Source: CAD feature listing. Evaluate the final solid. Frame: model axes, mm. A direction names the side the tool comes from. Give positions to 0.01 mm unless a question says otherwise; leave off trailing zeros. Loops run counter-clockwise (first coordinate to the right, second up) from the corner with the lowest first, then second, coordinate; pieces in that order, holes last. Notation, with made-up numbers: M 53.25,55.5 L 89.25,55.5 A15 ccw 89.25,59.5 Z; hole C 11,-4 d4. An arc over 180 degrees is marked long. Answer in a Markdown table with one row per item.
```python
from build123d import *

# Parameters (mm, degrees)
SKETCH3_W             = 20.066
SKETCH3_H             = 20.066
BOSS_EXTRUDE1_DEPTH   = 4.7625
SKETCH6_R             = 8.5725
CUT_EXTRUDE4_DEPTH    = 5.7625
SKETCH61_R            = 8.5725
CUT_EXTRUDE41_DEPTH   = 5.7625
SKETCH62_R            = 9.525
CUT_EXTRUDE42_DEPTH   = 5.7625
F_6_CLEARANCE_HOLE1_D = 4.3053
CUT_EXTRUDE43_REACH   = 6.763
FILLET1_R             = 1.5875


with BuildPart() as part:
    # Sketch3 → Boss-Extrude1 (new body)
    with BuildSketch(Plane.XY):
        with BuildLine():
            Line((-0.5715, -189.484), (41.8465, -189.484))
            ThreePointArc((41.8465, -189.484), (42.969032015, -189.019032015), (43.434, -187.8965))
            Line((43.434, -187.8965), (43.434, -183.134))
            ThreePointArc((43.434, -183.134), (45.293871939, -178.643871939), (49.784, -176.784))
            Line((49.784, -176.784), (54.5465, -176.784))
            ThreePointArc((54.5465, -176.784), (55.669032015, -176.319032015), (56.134, -175.1965))
            Line((56.134, -175.1965), (56.134, -72.4535))
            ThreePointArc((56.134, -72.4535), (55.669032015, -71.330967985), (54.5465, -70.866))
            Line((54.5465, -70.866), (49.784, -70.866))
            ThreePointArc((49.784, -70.866), (45.293871939, -69.006128061), (43.434, -64.516))
            Line((43.434, -64.516), (43.434, -59.7535))
            ThreePointArc((43.434, -59.7535), (42.969032015, -58.630967985), (41.8465, -58.166))
            Line((41.8465, -58.166), (32.3215, -58.166))
            ThreePointArc((32.3215, -58.166), (31.198967985, -57.701032015), (30.734, -56.5785))
            Line((30.734, -56.5785), (30.734, -13.7795))
            ThreePointArc((30.734, -13.7795), (30.269032015, -12.656967985), (29.1465, -12.192))
            Line((29.1465, -12.192), (-54.5465, -12.192))
            ThreePointArc((-54.5465, -12.192), (-55.669032015, -12.656967985), (-56.134, -13.7795))
            Line((-56.134, -13.7795), (-56.134, -140.9065))
            ThreePointArc((-56.134, -140.9065), (-55.669032015, -142.029032015), (-54.5465, -142.494))
            Line((-54.5465, -142.494), (-3.7465, -142.494))
            ThreePointArc((-3.7465, -142.494), (-2.623967985, -142.958967985), (-2.159, -144.0815))
            Line((-2.159, -144.0815), (-2.159, -187.8965))
            ThreePointArc((-2.159, -187.8965), (-1.694032015, -189.019032015), (-0.5715, -189.484))
        make_face()
        with Locations((23.8125, -158.75)):
            Rectangle(SKETCH3_W, SKETCH3_H, mode=Mode.SUBTRACT)
    extrude(amount=BOSS_EXTRUDE1_DEPTH)

    # Sketch6 → Cut-Extrude4 (cut, through all)
    with BuildSketch(Plane(origin=(161.486140968, -518.011138809, 4.7625), x_dir=(1, 0, 0), z_dir=(0, 0, 1))):
        with Locations((-137.673640968, 421.491138809)):
            Circle(SKETCH6_R)
    extrude(amount=-CUT_EXTRUDE4_DEPTH, mode=Mode.SUBTRACT)

    # Sketch61 → Cut-Extrude41 (cut, through all)
    with BuildSketch(Plane(origin=(147.833640968, -456.416138809, 4.7625), x_dir=(1, 0, 0), z_dir=(0, 0, 1))):
        with Locations((-137.673640968, 421.491138809)):
            Circle(SKETCH61_R)
    extrude(amount=-CUT_EXTRUDE41_DEPTH, mode=Mode.SUBTRACT)

    # Sketch62 → Cut-Extrude42 (cut, through all)
    with BuildSketch(Plane.XY.offset(4.7625)):
        with Locations((-37.592, -116.078)):
            Circle(SKETCH62_R)
    extrude(amount=-CUT_EXTRUDE42_DEPTH, mode=Mode.SUBTRACT)

    # #6 Clearance Hole1 (through all)
    with Locations(Plane(origin=(36.5125, -265.1125, 6.35), x_dir=(-1, 0, 0), z_dir=(0, 0, 1))):
        with Locations((49.4665, -130.4925), (-12.7, -136.525), (46.1645, -240.9825)):
            Hole(F_6_CLEARANCE_HOLE1_D / 2)

    # Sketch67 → Cut-Extrude43 (cut, up to next)
    with BuildSketch(Plane(origin=(0, 0, 0), x_dir=(-1, 0, 0), z_dir=(0, 0, -1)), mode=Mode.PRIVATE) as cut_extrude43_sk1:
        with BuildLine():
            Line((-19.558, -170.65625), (-19.558, -167.48125))
            ThreePointArc((-19.558, -167.48125), (-16.66875, -164.592), (-13.7795, -167.48125))
            Line((-13.7795, -167.48125), (-13.7795, -170.65625))
            ThreePointArc((-13.7795, -170.65625), (-16.66875, -173.5455), (-19.558, -170.65625))
        make_face()
    cut_extrude43_tool1 = extrude(cut_extrude43_sk1.sketch, amount=-CUT_EXTRUDE43_REACH, mode=Mode.PRIVATE) & part.part
    add(cut_extrude43_tool1.solids().sort_by_distance((16.66875, -169.06875, 0))[0], mode=Mode.SUBTRACT)
    # Sketch67 → Cut-Extrude43 (cut, up to next)
    with BuildSketch(Plane(origin=(0, 0, 0), x_dir=(-1, 0, 0), z_dir=(0, 0, -1)), mode=Mode.PRIVATE) as cut_extrude43_sk2:
        with BuildLine():
            Line((-28.067, -146.84375), (-28.067, -150.01875))
            ThreePointArc((-28.067, -150.01875), (-30.95625, -152.908), (-33.8455, -150.01875))
            Line((-33.8455, -150.01875), (-33.8455, -146.84375))
            ThreePointArc((-33.8455, -146.84375), (-30.95625, -143.9545), (-28.067, -146.84375))
        make_face()
    cut_extrude43_tool2 = extrude(cut_extrude43_sk2.sketch, amount=-CUT_EXTRUDE43_REACH, mode=Mode.PRIVATE) & part.part
    add(cut_extrude43_tool2.solids().sort_by_distance((30.95625, -148.43125, 0))[0], mode=Mode.SUBTRACT)

    # Fillet1
    fillet1_edges = [part.edges().sort_by_distance(p)[0] for p in [
        (33.8455, -168.783, 2.38125),
        (13.7795, -148.717, 2.38125),
    ]]
    fillet(fillet1_edges, radius=FILLET1_R)


solid = part.part
```
1) Pull-direction query (Y, two-part tool) for faces 1 (the flat face through (52, -176.784, 2)), 2 (the cylindrical face through (31.02, -143.955, 2.348)), 3 (the flat face through (37, -58.166, 2)), 4 (the flat face through (43.434, -62, 2)); classes: released by +Y, released by -Y, zero draft, split by the parting line, or undercut.
Reply:
| item | result |
|---|---|
| face 1 | released by -Y |
| face 2 | undercut |
| face 3 | released by +Y |
| face 4 | zero draft |
2) Pin query (flat end, axial travel): pin 1 Ø22.5 at (x, y) = (10.16, -34.925) entering from +Z; pin 2 Ø2.5 at (x, z) = (35, 2.5) entering from +Y; pin 3 Ø1.5 at (y, z) = (-169.5, 2) entering from -X; pin 4 Ø2.5 at (x, z) = (-33.5, 2) entering from -Y. Return the tip coordinate at first contact, or that it passes through.
Reply:
| item | result |
|---|---|
| pin 1 | stops at z = 4.76 |
| pin 2 | stops at y = -58.17 |
| pin 3 | stops at x = -2.16 |
| pin 4 | stops at y = -142.49 |
3) Material intervals for L1, parallel to X at y = -24.13, z = 2.6; L2, parallel to X at y = -96.52, z = 2.5 (3 decimals); L3, parallel to Y at x = 19, z = 3.5, sorted ascending.
Reply:
| item | result |
|---|---|
| L1 | x = -56.13 to -11.8, -7.5 to 30.73 |
| L2 | x = -56.134 to 15.24, 32.385 to 56.134 |
| L3 | y = -189.48 to -172.36, -148.72 to -103.61, -89.43 to -12.19 |
4) Section A-A, the plane x = 10.16. Return loops of the section in (y, z), then the cut area to 3 significant figures.
Reply:
| item | result |
|---|---|
| outline | M -189.48,0 L -43.5,0 L -43.5,4.76 L -189.48,4.76 Z; M -26.35,0 L -12.19,0 L -12.19,4.76 L -26.35,4.76 Z |
| area | 763 mm² |
5) Section B-B, the plane y = -24.13. Return loops of the section in (x, z), then the cut area to 3 significant figures.
Reply:
| item | result |
|---|---|
| outline | M -56.13,0 L -11.8,0 L -11.8,4.76 L -56.13,4.76 Z; M -7.5,0 L 30.73,0 L 30.73,4.76 L -7.5,4.76 Z |
| area | 393 mm² |
6) Section C-C, the plane x = 22. Return loops of the section in (y, z), then the cut area to 3 significant figures.
Reply:
| item | result |
|---|---|
| outline | M -189.48,0 L -168.78,0 L -168.78,4.76 L -189.48,4.76 Z; M -148.72,0 L -104.9,0 L -104.9,4.76 L -148.72,4.76 Z; M -88.14,0 L -12.19,0 L -12.19,4.76 L -88.14,4.76 Z |
| area | 669 mm² |
7) Set-up query: faces 5 (the flat face through (43.434, -186, 2)), 6 (the flat face through (-2.159, -166, 2)), 7 (the flat face through (-1, -100, 4.762)), 8 (the flat face through (22, -148.717, 2)). Return all of +Z, -Z, +X, -X, +Y, -Y with unobstructed straight access to the full face (end or side cutting, diameter ignored); none if empty.
Reply:
| item | result |
|---|---|
| face 5 | +Z, -Z, +X, -Y |
| face 6 | +Z, -Z, -X, -Y |
| face 7 | +Z, +X, -X, +Y, -Y |
| face 8 | +Z, -Z |
8) Section D-D, the plane z = 1.55. Count the separate pieces of the cut face and the enclosed holes in it, then the cut area to 3 significant figures.
Reply:
| item | result |
|---|---|
| separate pieces | 1 |
| enclosed holes | 7 |
| area | 14,700 mm² |
